Design review of the part built by this model. Coordinates are the model's own, in mm. Give positions to 0.01 mm unless a question says otherwise; leave off trailing zeros. Write each loop counter-clockwise with the first axis right and the second up, starting at its lowest first coordinate (ties: lowest second). Pieces come first, ordered by that corner, then holes. Notation, with made-up numbers: M -31,43.25 L 16,43.25 A14 cw 16,57.25 Z; hole C -4,36 d10. An arc over 180 degrees is marked long. Write each question's results on one line, items separated by ' | '. Start each with the question number.
from build123d import *

# Parameters (mm, degrees)
SKETCH1_W           = 162
SKETCH1_H           = 50
SKETCH1_R           = 10
SKETCH1_R_2         = 2
BOSS_EXTRUDE1_DEPTH = 10


with BuildPart() as part:
    # Sketch1 → Boss-Extrude1 (new body)
    with BuildSketch(Plane(origin=(0, 0, 0), x_dir=(0, 0, -1), z_dir=(1, 0, 0))):
        Rectangle(SKETCH1_W, SKETCH1_H)
        Circle(SKETCH1_R, mode=Mode.SUBTRACT)
        with Locations((-68.5, 10)):
            Circle(SKETCH1_R_2, mode=Mode.SUBTRACT)
        with Locations((-68.5, -10)):
            Circle(SKETCH1_R_2, mode=Mode.SUBTRACT)
        with Locations((68.5, 10)):
            Circle(SKETCH1_R_2, mode=Mode.SUBTRACT)
        with Locations((68.5, -10)):
            Circle(SKETCH1_R_2, mode=Mode.SUBTRACT)
    extrude(amount=BOSS_EXTRUDE1_DEPTH)


solid = part.part
Q1. Wall thickness on line 1 along Y through (x, z) = (4.75, 68.5); line 2 along Y through (x, z) = (2.5, 67); line 3 along Z through (x, y) = (3.25, -6): over which ranges is each line inside the solid? List them lowest first. Write a range as from..to.
Q2. We need section A-A on z = 0. Write out the cut boundary in (x, y), and give its area (3 significant figures).
Q3. We need section D-D on z = 68.5. Write out the cut boundary in (x, y), and give its area (3 significant figures).
Q4. The part is to be moulded in two halves that separate along Z. For faces 1 (the cylindrical face through (4.93, -9.76, 2.17)), 2 (the flat face through (5, 0, -81)), 3 (the flat face through (5, 0, 81)), say which applies: pulls with the +Z half, pulls with the -Z half, needs draft (parallel to the pull), parting line crosses it, or undercut.
Q5. We need section B-B on y = 0. Write out the cut boundary in (x, z).
Q6. We need section C-C on x = 5.25. Write out the cut boundary in (y, z), and give its area (3 significant figures).
Answer sheet:
1) line 1: -25..-12, -8..8, 12..25 | line 2: -25..-11.32, -8.68..8.68, 11.32..25 | line 3: -81..-8, 8..81
2) outline: M 0,-25 L 10,-25 L 10,-10 L 0,-10 Z; M 0,10 L 10,10 L 10,25 L 0,25 Z | area: 300 mm^2
3) outline: M 0,-25 L 10,-25 L 10,-12 L 0,-12 Z; M 0,-8 L 10,-8 L 10,8 L 0,8 Z; M 0,12 L 10,12 L 10,25 L 0,25 Z | area: 420 mm^2
4) face 1: undercut | face 2: pulls with the -Z half | face 3: pulls with the +Z half
5) outline: M 0,-81 L 10,-81 L 10,-10 L 0,-10 Z; M 0,10 L 10,10 L 10,81 L 0,81 Z
6) outline: M -25,-81 L 25,-81 L 25,81 L -25,81 Z; hole C -10,-68.5 d4; hole C -10,68.5 d4; hole C 0,0 d20; hole C 10,-68.5 d4; hole C 10,68.5 d4 | area: 7,740 mm^2
